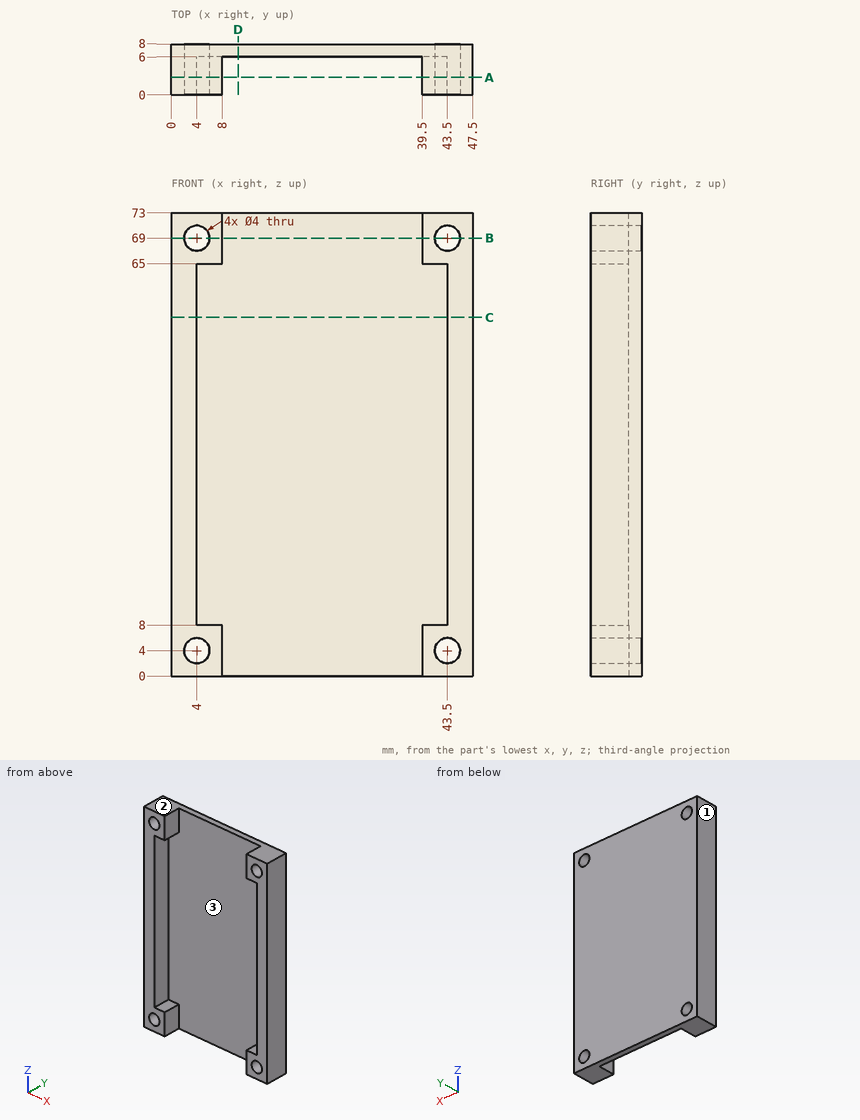
Part print with two shaded views. Sizes in mm from the minimum x, y, z corner. Round coordinates to 2 decimals unless told otherwise and drop trailing zeros. Write each loop counter-clockwise with the first axis right and the second up, starting at its lowest first coordinate (ties: lowest second). Pieces come first, ordered by that corner, then holes. Notation, with made-up numbers: (31.25, 75.5) -> (35.25, 75.5) arc R16 ccw to (35.25, 98.5) -> close; hole circle Ø2 at (2, 24). An arc over 180 degrees is marked (long way). Put each result on its own line as item: value.
Item 1: Slice it at D-D, the plane x = 10.5. Give the cut face in (y, z).
Here are the results:
outline: (6, 0) -> (8, 0) -> (8, 73) -> (6, 73) -> close
Item 2: Two-plate mould, pull along X, no slides. Class the marked faces 1, 2 and 3: pulls with the +X half, pulls with the -X half, needs draft (parallel to the pull), parting line crosses it, or undercut.
Here are the results:
face 1: pulls with the -X half
face 2: needs draft
face 3: undercut
Item 3: Flat gauge pins, fed straight in: P1, Ø3, axis at x = 24.5, y = 3.5, coming from the -Z side; P2, Ø5, axis at x = 28.5, z = 33, coming from the -Y side. Where does each tip first touch, or does it go through?
Here are the results:
P1: passes through
P2: stops at y = 6
Item 4: Slice it at B-B, the plane z = 69. Give the cut face in (x, y), plus the area to 3 significant figures.
Here are the results:
outline: (0, 0) -> (2, 0) -> (2, 8) -> (0, 8) -> close; (6, 0) -> (8, 0) -> (8, 6) -> (39.5, 6) -> (39.5, 0) -> (41.5, 0) -> (41.5, 8) -> (6, 8) -> close; (45.5, 0) -> (47.5, 0) -> (47.5, 8) -> (45.5, 8) -> close
area: 127 mm^2
Item 5: Slice it at A-A, the plane y = 2.75. Give the cut face in (x, z), plus the area to 3 significant figures.
Here are the results:
outline: (0, 0) -> (8, 0) -> (8, 8) -> (4, 8) -> (4, 65) -> (8, 65) -> (8, 73) -> (0, 73) -> close; (39.5, 0) -> (47.5, 0) -> (47.5, 73) -> (39.5, 73) -> (39.5, 65) -> (43.5, 65) -> (43.5, 8) -> (39.5, 8) -> close; hole circle Ø4 at (4, 4); hole circle Ø4 at (4, 69); hole circle Ø4 at (43.5, 4); hole circle Ø4 at (43.5, 69)
area: 662 mm^2
Item 6: Wall check: probe 1 along X at (y, z) = (6.25, 4); probe 2 along X at (y, z) = (3.75, 4); probe 3 along Z at (x, y) = (4, 6.5). Give the ranges that are in metal, low to high. Write a range as from..to.
Here are the results:
probe 1: x = 0..2, 6..41.5, 45.5..47.5
probe 2: x = 0..2, 6..8, 39.5..41.5, 45.5..47.5
probe 3: z = 0..2, 6..67, 71..73
Item 7: Slice it at C-C, the plane z = 56.5. Give the cut face in (x, y).
Here are the results:
outline: (0, 0) -> (4, 0) -> (4, 6) -> (43.5, 6) -> (43.5, 0) -> (47.5, 0) -> (47.5, 8) -> (0, 8) -> close
